Autodesk Fusion 360 part; units mm, degrees
sketch "Top" plane through (0, 0, 0) normal (0, 1, 0) x (1, 0, 0)
  line L0 (-17, 0) -> (118, 0) construction
  circle A0 centre (0, 0) radius 5
  circle A1 centre (29.5, 0) radius 5
  line L1 (-17, 7.5) -> (57, 7.5)
  line L2 (57, 7.5) -> (57, -7.5)
  line L3 (57, -7.5) -> (-17, -7.5)
  line L4 (-17, -7.5) -> (-17, 7.5)
  line L5 (57, 32) -> (25, 32)
  line L6 (25, 32) -> (25, -32)
  line L7 (25, -32) -> (57, -32)
  line L8 (57, -32) -> (57, 32)
  line L9 (25, 32) -> (18, 7.5)
  line L10 (25, -32) -> (18, -7.5)
  circle A2 centre (14.5, 0) radius 2.413
  circle A3 centre (50.5, 0) radius 2.413
  point P0 (-17, 0)
  point P1 (57, 0)
  point P2 (57, 0)
  dimension "d1" = 10
  dimension "d2" = 10
  dimension "d3" = 29.5
  dimension "d4" = 74
  dimension "d5" = 15
  dimension "d6" = 17
  dimension "d7" = 64
  dimension "d8" = 18
  dimension "d9" = 32
  dimension "d16" = 4.826
  dimension "d17" = 14.5
  dimension "d18" = 4.826
  dimension "d19" = 50.5
extrude "Extrude1" add sketch "Top" along normal blind 3 contours A1 L1 L2 L3 L6 L8 | A1 L1 L3 L4 L6 | L1 L5 L6 L8 | L1 L6 L9 | L3 L6 L10 | L3 L6 L7 L8 | A2 | A3
fillet "Fillet1" radius 1 6 edges at (-17, 1.5, 7.5) (-17, 1.5, -7.5) (57, 1.5, 32) (57, 1.5, -32) (25, 1.5, -32) (25, 1.5, 32)
fillet "Fillet2" radius 4 2 edges at (18, 1.5, -7.5) (18, 1.5, 7.5)
extrude "Extrude2" add sketch "Top" along normal blind 3 from surface at 3 contours A2 | A3
fillet "Fillet3" radius 1 2 edges at (12.2503, 6, 0.8726) (48.2503, 6, 0.8726)
For this review, take the finished solid that the model builds, in its own axes (mm). A direction names the side the tool comes from. Give positions to 0.01 mm unless a question says otherwise; leave off trailing zeros. Loops run counter-clockwise (first coordinate to the right, second up) from the corner with the lowest first, then second, coordinate; pieces in that order, holes last.
Item 1: For line 1 along X through (y, z) = (1.65, 0); line 2 along Z through (x, y) = (29.5, 1.85); line 3 along X through (y, z) = (2.2, -3.5), list the stretches that pass through material, from the lowest coordinate up.
Item 2: Take a section at B-B, the plane z = 0. State the section outline as (x, y) points, and give its area (3 significant figures).
Item 3: Take a section at D-D, the plane x = 50.5. State the section outline as (y, z) points.
Item 4: Take a section at A-A, the plane x = 0. State the section outline as (y, z) points, and give its area (3 significant figures).
Item 5: Take a section at C-C, the plane y = 4.1. State the section outline as (x, z) points, and give its area (3 significant figures).
Item 6: Tool access review of faces 1 (the flat face through (-1, 1, -7.5)), 2 (the cylindrical face through (12.09, 3.99, 0.11)), 3 (the flat face through (0, 1, 7.5)): name each direction out of +Z, -Z, +X, -X, +Y, -Y from which nothing blocks a thin tool from reaching the whole face with its end or side.
Item 7: Insertion check: pin 1 (10 mm diameter, centred on x = 22, z = 13.5, fed in from +Y); pin 2 (1.5 mm diameter, centred on x = -1.5, y = 2, fed in from +Z); pin 3 (2 mm diameter, centred on x = 2.5, y = 5, fed in from +Z); pin 4 (2.5 mm diameter, centred on x = -1, y = 2, fed in from -Z). Each pin has a flat end and moves straight along its axis. Give the tip position at first contact, or say it passes through.
Calculated:
1. line 1: x = -17 to -5, 5 to 24.5, 34.5 to 57
1. line 2: z = -32 to -5, 5 to 32
1. line 3: x = -17 to -3.57, 3.57 to 25.93, 33.07 to 57
2. outline: (-17, 0) - (-5, 0) - (-5, 3) - (-17, 3) - close; (5, 0) - (24.5, 0) - (24.5, 3) - (16.91, 3) - (16.91, 5) arc R1 ccw to (15.91, 6) - (13.09, 6) arc R1 ccw to (12.09, 5) - (12.09, 3) - (5, 3) - close; (34.5, 0) - (57, 0) - (57, 3) - (52.91, 3) - (52.91, 5) arc R1 ccw to (51.91, 6) - (49.09, 6) arc R1 ccw to (48.09, 5) - (48.09, 3) - (34.5, 3) - close
2. area: 190 mm2
3. outline: (0, -32) - (3, -32) - (3, -2.41) - (5, -2.41) arc R1 ccw to (6, -1.41) - (6, 1.41) arc R1 ccw to (5, 2.41) - (3, 2.41) - (3, 32) - (0, 32) - close
4. outline: (0, -7.5) - (3, -7.5) - (3, -5) - (0, -5) - close; (0, 5) - (3, 5) - (3, 7.5) - (0, 7.5) - close
4. area: 15.0 mm2
5. outline: circle Ø4.83 at (14.5, 0); circle Ø4.83 at (50.5, 0)
5. area: 36.6 mm2
6. face 1: -Z, -X, +Y, -Y
6. face 2: +Y
6. face 3: +Z, -X, +Y, -Y
7. pin 1: stops at y = 3
7. pin 2: stops at z = 7.5
7. pin 3: passes through
7. pin 4: stops at z = -7.5
